Geometry: final body of the model. Coordinates: model frame, mm. A direction names the side the tool comes from. Round coordinates to 2 decimals unless told otherwise and drop trailing zeros. Order: outer loops, then holes, each group sorted by start corner. A loop starts at its lowest first (then second) coordinate and runs counter-clockwise, first axis right, second up. Notation, with made-up numbers: (55.5, 46.5) -> (103.5, 46.5) arc R26 ccw to (103.5, 81.5) -> close; hole circle Ø5 at (-18.75, 76.25). An arc over 180 degrees is marked (long way). Put each result on its own line as item: value.
```python
from build123d import *

# Parameters (mm, degrees)
SM_BASE_FLANGE_1_DEPTH = 50
SKETCH_6_R             = 6.9
CUT_EXTRUDE_1_DEPTH    = 10
SKETCH_7_R             = 6.9
CUT_EXTRUDE_2_DEPTH    = 10
OTHER_START            = 20.788939367
OTHER_1_OUTLINE_W      = 10
OTHER_1_OUTLINE_H      = 8
OTHER_1_DEPTH          = 3.535533906
OTHER_START_2          = 56.144278426
OTHER_1_2_OUTLINE_W    = 38
OTHER_1_2_OUTLINE_H    = 8
OTHER_1_2_DEPTH        = 3.535533906
OTHER_1_3_OUTLINE_W    = 7
OTHER_1_3_OUTLINE_H    = 10
OTHER_1_3_DEPTH        = 3.535533906
OTHER_START_3          = -35.355339059
OTHER_1_4_OUTLINE_W    = 7
OTHER_1_4_OUTLINE_H    = 38
OTHER_1_4_DEPTH        = 3.535533906


# Read off the part's stored shape, not the designer's step: Затупленный угол1
# Sheet-metal steps are written as plain solids
with BuildPart() as part:
    # Sketch 1 → Базовая кромка1 (new body)
    with BuildSketch(Plane.XY):
        with BuildLine():
            Line((34.4, 308.5), (-9.6, 308.5))
            ThreePointArc((-9.6, 308.5), (-16.671067812, 305.571067812), (-19.6, 298.5))
            Line((-19.6, 298.5), (-19.6, 254.005167492))
            ThreePointArc((-19.6, 254.005167492), (-19.58726466, 253.500643348), (-19.549091078, 252.997404261))
            Line((-19.549091078, 252.997404261), (-0.076363384, 60.753893608))
            ThreePointArc((-0.076363384, 60.753893608), (-0.01910301, 59.999034978), (0, 59.242248762))
            Line((0, 59.242248762), (0, 0))
            Line((0, 0), (-5, 0))
            Line((-5, 0), (-5, 59.242248762))
            ThreePointArc((-5, 59.242248762), (-5.01273534, 59.746772906), (-5.050908922, 60.250011993))
            Line((-5.050908922, 60.250011993), (-24.523636616, 252.493522646))
            ThreePointArc((-24.523636616, 252.493522646), (-24.58089699, 253.248381276), (-24.6, 254.005167492))
            Line((-24.6, 254.005167492), (-24.6, 298.5))
            ThreePointArc((-24.6, 298.5), (-20.206601718, 309.106601718), (-9.6, 313.5))
            Line((-9.6, 313.5), (34.4, 313.5))
            Line((34.4, 313.5), (34.4, 308.5))
        make_face()
    extrude(amount=SM_BASE_FLANGE_1_DEPTH)

    # Эскиз6 → Вырез-Вытянуть1 (cut)
    with BuildSketch(Plane.ZY.offset(5)):
        with Locations(Location((25, 15, 0), (0, 0, 270))):
            Circle(SKETCH_6_R)
        with Locations(Location((25, 40, 0), (0, 0, 270))):
            Circle(SKETCH_6_R)
    extrude(amount=-CUT_EXTRUDE_1_DEPTH, mode=Mode.SUBTRACT)

    # Эскиз7 → Вырез-Вытянуть2 (cut)
    with BuildSketch(Plane(origin=(0, 313.5, 0), x_dir=(1, 0, 0), z_dir=(0, 1, 0))):
        with Locations(Location((9.4, -25, 0), (0, 0, 180))):
            Circle(SKETCH_7_R)
    extrude(amount=-CUT_EXTRUDE_2_DEPTH, mode=Mode.SUBTRACT)

    # Other 1 outline → Other 1 (cut)
    with BuildSketch(Plane(origin=(0, 0, 0), x_dir=(0.707106781186548, 0, 0.707106781186547), z_dir=(0.707106781186547, 0, -0.707106781186548)).offset(OTHER_START)):
        with Locations((24, -311)):
            Rectangle(OTHER_1_OUTLINE_W, OTHER_1_OUTLINE_H)
    extrude(amount=OTHER_1_DEPTH, mode=Mode.SUBTRACT)

    # Other 1 2 outline → Other 1 2 (cut)
    with BuildSketch(Plane(origin=(0, 0, 0), x_dir=(0.707106781186548, 0, -0.707106781186547), z_dir=(0.707106781186547, 0, 0.707106781186548)).offset(OTHER_START_2)):
        with Locations((3, 311)):
            Rectangle(OTHER_1_2_OUTLINE_W, OTHER_1_2_OUTLINE_H)
    extrude(amount=OTHER_1_2_DEPTH, mode=Mode.SUBTRACT)

    # Other 1 3 outline → Other 1 3 (cut)
    with BuildSketch(Plane(origin=(0, 0, 0), x_dir=(1, 0, 0), z_dir=(0, 0.7071067811865476, 0.7071067811865476))):
        with Locations((-2.5, 0)):
            Rectangle(OTHER_1_3_OUTLINE_W, OTHER_1_3_OUTLINE_H)
    extrude(amount=OTHER_1_3_DEPTH, mode=Mode.SUBTRACT)

    # Other 1 4 outline → Other 1 4 (cut)
    with BuildSketch(Plane(origin=(0, 0, 0), x_dir=(1, 0, 0), z_dir=(0, 0.7071067811865476, -0.7071067811865476)).offset(OTHER_START_3)):
        with Locations((-2.5, -21)):
            Rectangle(OTHER_1_4_OUTLINE_W, OTHER_1_4_OUTLINE_H)
    extrude(amount=OTHER_1_4_DEPTH, mode=Mode.SUBTRACT)


solid = part.part
```
1. Set-up query: faces 1 (the face through (-19.6, 277, 25)), 2 (the face through (-5, 29, 25)), 3 (the face through (0, 30, 25)), 4 (the face through (-2, 0, 25)). Return all of +Z, -Z, +X, -X, +Y, -Y with unobstructed straight access to the full face (end or side cutting, diameter ignored); none if empty.
Ans:
face 1: +Z, -Z, +X
face 2: +Z, -Z, -X, -Y
face 3: +Z, -Z, +X, -Y
face 4: +Z, -Z, +X, -X, -Y
2. Cut plane B-B on x = 9.4. Return loops of the section in (y, z), and give its area (3 significant figures).
Ans:
outline: (308.5, 0) -> (313.5, 0) -> (313.5, 18.1) -> (308.5, 18.1) -> close; (308.5, 31.9) -> (313.5, 31.9) -> (313.5, 50) -> (308.5, 50) -> close
area: 181 mm²
3. Cut plane D-D on z = 11.5. Return loops of the section in (x, y), and give its area (3 significant figures).
Ans:
outline: (-24.6, 254.01) arc R15 ccw to (-24.52, 252.49) -> (-5.05, 60.25) arc R10 cw to (-5, 59.24) -> (-5, 0) -> (0, 0) -> (0, 59.24) arc R15 ccw to (-0.08, 60.75) -> (-19.55, 253) arc R10 cw to (-19.6, 254.01) -> (-19.6, 298.5) arc R10 cw to (-9.6, 308.5) -> (34.4, 308.5) -> (34.4, 313.5) -> (-9.6, 313.5) arc R15 ccw to (-24.6, 298.5) -> close
area: 1,820 mm²
4. Cut plane C-C on y = 15. Return loops of the section in (x, z).
Ans:
outline: (-5, 0) -> (0, 0) -> (0, 18.1) -> (-5, 18.1) -> close; (-5, 31.9) -> (0, 31.9) -> (0, 50) -> (-5, 50) -> close
5. Contact query for flat-ended pins moving along their axis: P1, Ø22, axis at y = 40, z = 25, coming from the -X side; P2, Ø6, axis at x = -1, y = 128.5, coming from the -Z side; P3, Ø22, axis at y = 273.5, z = 18, coming from the +X side; P4, Ø10, axis at y = 88, z = 12, coming from the +X side. Output: stop coordinate, or through.
Ans:
P1: x = -5
P2: through
P3: x = -19.6
P4: x = -2.33
6. Material intervals for probe 1 along Z at (x, y) = (-2, 15); probe 2 along X at (y, z) = (253, 42.5); probe 3 along X at (y, z) = (42.5, 9), sorted ascending.
Ans:
probe 1: 0 to 18.1, 31.9 to 50
probe 2: -24.57 to -19.55
probe 3: -5 to 0
7. Draft query along Y for faces 5 (the face through (-3, 2, 47)), 6 (the face through (-2.535, 45.476, 20.801)), 7 (the face through (34.4, 311, 25)). Return one class per face: +Y half, -Y half, draft (parallel to the pull), parting line (faces both ways), or undercut.
Ans:
face 5: -Y half
face 6: undercut
face 7: draft
8. Cut plane A-A on z = 25. Return loops of the section in (x, y).
Ans:
outline: (-24.6, 254.01) arc R15 ccw to (-24.52, 252.49) -> (-5.05, 60.25) arc R10 cw to (-5, 59.24) -> (-5, 46.9) -> (0, 46.9) -> (0, 59.24) arc R15 ccw to (-0.08, 60.75) -> (-19.55, 253) arc R10 cw to (-19.6, 254.01) -> (-19.6, 298.5) arc R10 cw to (-9.6, 308.5) -> (2.5, 308.5) -> (2.5, 313.5) -> (-9.6, 313.5) arc R15 ccw to (-24.6, 298.5) -> close; (-5, 0) -> (0, 0) -> (0, 8.1) -> (-5, 8.1) -> close; (-5, 21.9) -> (0, 21.9) -> (0, 33.1) -> (-5, 33.1) -> close; (16.3, 308.5) -> (34.4, 308.5) -> (34.4, 313.5) -> (16.3, 313.5) -> close
